```python
from build123d import *

# Parameters (mm, degrees)
SKETCH_1_R          = 45
EXTRUDE_1_DEPTH     = 1
SKETCH_2_R          = 1
CUT_EXTRUDE_1_DEPTH = 64.647466564
SKETCH_4_R          = 4
CUT_EXTRUDE_2_DEPTH = 64.647466564
SKETCH_5_W          = 0.7
SKETCH_5_H          = 28.5
EXTRUDE_2_DEPTH     = 12
EXTRUDE_2_2_DEPTH   = 3.5
EXTRUDE_3_DEPTH     = 12


with BuildPart() as part:
    # 草图1 → 凸台-拉伸1 (new body)
    with BuildSketch(Plane.XY):
        Circle(SKETCH_1_R)
    extrude(amount=EXTRUDE_1_DEPTH)

    # 草图2 → 切除-拉伸1 (cut, through all)
    with BuildSketch(Plane.XY.offset(1)):
        with Locations((20, -16.5)):
            Circle(SKETCH_2_R)
        with Locations((20, 16.5)):
            Circle(SKETCH_2_R)
        with Locations((-20, 16.5)):
            Circle(SKETCH_2_R)
        with Locations((-20, -16.5)):
            Circle(SKETCH_2_R)
        with Locations((10, -16.5)):
            Circle(SKETCH_2_R)
        with Locations((10, 16.5)):
            Circle(SKETCH_2_R)
        with Locations((-10, 16.5)):
            Circle(SKETCH_2_R)
        with Locations((-10, -16.5)):
            Circle(SKETCH_2_R)
    extrude(amount=-CUT_EXTRUDE_1_DEPTH, mode=Mode.SUBTRACT)

    # 草图4 → 切除-拉伸2 (cut, through all)
    with BuildSketch(Plane.XY.offset(1)):
        Circle(SKETCH_4_R)
    extrude(amount=-CUT_EXTRUDE_2_DEPTH, mode=Mode.SUBTRACT)

    # 草图5 → Extrude 2 (add)
    with BuildSketch(Plane.XY.offset(1)):
        with Locations((16.331438859, -0.213782194)):
            Rectangle(SKETCH_5_W, SKETCH_5_H)
    extrude(amount=EXTRUDE_2_DEPTH)

    # 草图9 → Extrude 2 2 (add)
    with BuildSketch(Plane.XY.offset(1)):
        Polygon((16.681438859, 14.736217806), (-16.018561141, 14.736217806), (-16.018561141, 14.036217806), (15.981438859, 14.036217806), (16.681438859, 14.036217806), align=None)
    extrude(amount=EXTRUDE_2_2_DEPTH)

    # 草图10 → 凸台-拉伸3 (add)
    with BuildSketch(Plane.XY.offset(1)):
        Polygon((16.681438859, -14.463782194), (16.681438859, -15.163782194), (-16.718561141, -15.163782194), (-16.718561141, 14.736217806), (-16.018561141, 14.736217806), (-16.018561141, -14.463782194), (15.981438859, -14.463782194), align=None)
    extrude(amount=EXTRUDE_3_DEPTH)


solid = part.part
```
Geometry check sheet. Reference: the model listing, model coordinates, mm. A direction names the side the tool comes from. Give positions to 0.01 mm unless a question says otherwise; leave off trailing zeros. Loops run counter-clockwise (first coordinate to the right, second up) from the corner with the lowest first, then second, coordinate; pieces in that order, holes last. Notation, with made-up numbers: M 62.5,76 L 67.5,76 A31 cw 67.5,110 Z; hole C -10.5,71.5 d6. An arc over 180 degrees is marked long. Write item = value, one per line.
(1) Sectioned sample at D-D, the plane z = 10.25. Record the cut outline in (x, y).
Answer below:
outline = M -16.72,-15.16 L 16.68,-15.16 L 16.68,14.04 L 15.98,14.04 L 15.98,-14.46 L -16.02,-14.46 L -16.02,14.74 L -16.72,14.74 Z
(2) Sectioned sample at C-C, the plane z = 2.5. Record the cut outline in (x, y), plus the area to 3 significant figures.
Answer below:
outline = M -16.72,-15.16 L 16.68,-15.16 L 16.68,14.74 L -16.72,14.74 Z; hole M -16.02,-14.46 L 15.98,-14.46 L 15.98,14.04 L -16.02,14.04 Z
area = 86.7 mm2
(3) Release check for a two-part mould opening along Y. For faces 4 (the face through (-16.719, 0, 7)), 5 (the face through (9.783, -17.476, 0.507)), 6 (the face through (0, -15.164, 7)) record: released by +Y, released by -Y, zero draft, split by the parting line, or undercut.
Answer below:
face_4 = zero draft
face_5 = undercut
face_6 = released by -Y
(4) Sectioned sample at A-A, the plane x = 0. Record the cut outline in (y, z), plus the area to 4 significant figures.
Answer below:
outline = M -45,0 L -4,0 L -4,1 L -14.46,1 L -14.46,13 L -15.16,13 L -15.16,1 L -45,1 Z; M 4,0 L 45,0 L 45,1 L 14.74,1 L 14.74,4.5 L 14.04,4.5 L 14.04,1 L 4,1 Z
area = 92.85 mm2
(5) Tool access check on faces 1 (the face through (0, 14.036, 3)), 2 (the face through (16.681, 0, 7)), 3 (the face through (0, -15, 13)). Record the directions out of +Z, -Z, +X, -X, +Y, -Y that give a thin tool (end or side, any length) a straight path to the whole face; none if there is none.
Answer below:
face_1 = +Z
face_2 = +Z, +X, +Y, -Y
face_3 = +Z, +X, -X, +Y, -Y
(6) Sectioned sample at B-B, the plane y = 2. Record the cut outline in (x, z).
Answer below:
outline = M -44.96,0 L -3.46,0 L -3.46,1 L -16.02,1 L -16.02,13 L -16.72,13 L -16.72,1 L -44.96,1 Z; M 3.46,0 L 44.96,0 L 44.96,1 L 16.68,1 L 16.68,13 L 15.98,13 L 15.98,1 L 3.46,1 Z
(7) Material ranges on line 1 (X direction, y = 8, z = 2); line 2 (Y direction, x = -10, z = 0.65); line 3 (Y direction, x = -20, z = 0.3), recorded low to high. Write a range as [from, to].
Answer below:
line_1 = [-16.72, -16.02], [15.98, 16.68]
line_2 = [-43.87, -17.5], [-15.5, 15.5], [17.5, 43.87]
line_3 = [-40.31, -17.5], [-15.5, 15.5], [17.5, 40.31]
(8) Gauge pin test, flat ends, axial feed: pin 1 Ø12 at (x, y) = (14, 26) entering from +Z; pin 2 Ø3.5 at (y, z) = (4.5, 7.5) entering from +X; pin 3 Ø6 at (y, z) = (3, 2.5) entering from -X. Record the tip position at first contact, or that the pin passes through.
Answer below:
pin_1 = 1
pin_2 = 16.68
pin_3 = -45
